CAD build for the part. Positions are in the model's coordinates, mm. Face numbers are marked on the shaded views. Round coordinates to 2 decimals unless told otherwise and drop trailing zeros. Write each loop counter-clockwise with the first axis right and the second up, starting at its lowest first coordinate (ties: lowest second). Pieces come first, ordered by that corner, then holes. Notation, with made-up numbers: (49, -23) -> (98, -23) arc R8 cw to (98, -19) -> close; hole circle Ø11 at (6.25, 66.5). An arc over 180 degrees is marked (long way). Put each result on its own line as item: value. Start each with the question number.
1. Flat gauge pins, fed straight in: P1, Ø3, axis at x = 16.5, z = 87, coming from the -Y side; P2, Ø2, axis at x = 6.5, z = -52.5, coming from the +Y side; P3, Ø12, axis at x = 26, y = 10.5, coming from the +Z side; P4, Ø6, axis at x = 16, y = 19, coming from the +Z side. Where does each tip first touch, or does it go through?
2. Pull direction Z, two halves, no side cores. Call the marked faces 1, 2 and 3: pulls with the +Z half, pulls with the -Z half, needs draft (parallel to the pull), parting line crosses it, or undercut.
3. Saw through at B-B on z = -102.5. List the corners of the cut face in (x, y), and give its area (3 significant figures).
4. Drill centre lines: line 1 (Z direction, x = 7.5, y = 12); line 2 (Z direction, x = 6.5, y = 21.5); line 3 (Z direction, x = 31, y = 3.5). Where is each one in solid material? Low to high. Write a range as from..to.
from build123d import *

# Parameters (mm, degrees)
BOSS_EXTRUDE1_DEPTH = 40
FILLET1_R           = 10
FILLET2_R           = 10


with BuildPart() as part:
    # Sketch2 → Boss-Extrude1 (new body)
    with BuildSketch(Plane(origin=(0, 0, 0), x_dir=(0, 0, -1), z_dir=(1, 0, 0))):
        Polygon((-160, 10), (-160, 20), (-180, 20), (-180, -20), (-160, -20), (-160, -10), (160, -10), (160, -20), (180, -20), (220, -20), (220, 40), (200, 40), (200, -10), (180, -10), (180, 40), (160, 40), (160, 10), align=None)
    extrude(amount=BOSS_EXTRUDE1_DEPTH)

    # Fillet1
    fillet1_edges = [part.edges().sort_by_distance(p)[0] for p in [
        (20, 20, 180),
        (20, 20, 160),
    ]]
    fillet(fillet1_edges, radius=FILLET1_R - 0.0001)  # a hair under: the kernel refuses the full size

    # Fillet2
    fillet2_edges = [part.edges().sort_by_distance(p)[0] for p in [
        (20, 40, -160),
        (20, 40, -220),
    ]]
    fillet(fillet2_edges, radius=FILLET2_R)


solid = part.part
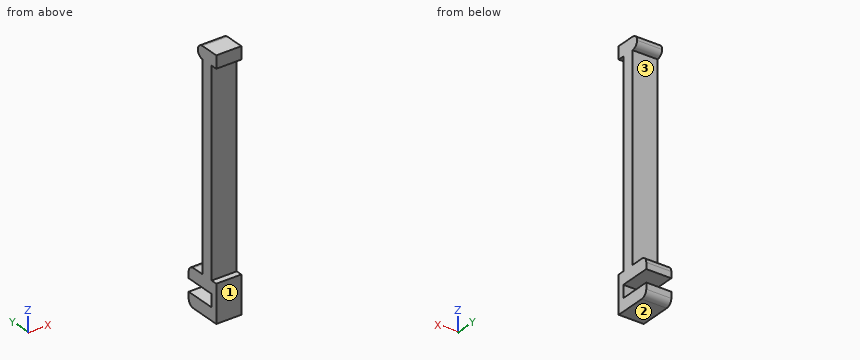
Return value:
1. P1: stops at y = -10
1. P2: stops at y = 10
1. P3: stops at z = 180
1. P4: stops at z = 178
2. face 1: needs draft
2. face 2: pulls with the -Z half
2. face 3: undercut
3. outline: (0, -10) -> (40, -10) -> (40, 10) -> (0, 10) -> close
3. area: 800 mm^2
4. line 1: z = -220..-200, -180..-160, 160.2..179.8
4. line 2: z = -220..-200, -180..-160
4. line 3: z = -220..-200, -180..180
